Here's how the part is built. I have some questions about the finished solid (model axes, mm). A direction names the side the tool comes from. Round coordinates to 2 decimals unless told otherwise and drop trailing zeros. Order: outer loops, then holes, each group sorted by start corner. A loop starts at its lowest first (then second) coordinate and runs counter-clockwise, first axis right, second up. Notation, with made-up numbers: (44.25, 32.5) -> (51.25, 32.5) arc R19 cw to (51.25, 61.5) -> close; hole circle Ø8 at (-14.5, 86.5). An arc over 180 degrees is marked (long way). Use a Markdown table: item, result. Add a question column.
(1) On a 3-axis mill with a long thin cutter (end or side, diameter ignored), from which of +Z, -Z, +X, -X, +Y, -Y can I reach the whole of each face in a straight line? I mean faces 1 (the face through (0, 3.3, -5.2)), 2 (the face through (1, 3.4, -1)), 3 (the face through (1, 3, 1)). Say none if no direction works.
(2) I'm going to push flat-ended pins straight in: P1, Ø1.7, axis at x = -1, z = -6.5, coming from the -Y side; P2, Ø4, axis at x = 0, z = 0, coming from the +Y side; P3, Ø2.5, axis at x = -0.5, z = 0, coming from the -Y side; P4, Ø1.5, axis at y = 0.5, z = -5.5, coming from the -X side. Where does each tip first touch, or does it pass through?
(3) I want a section at B-B, the plane z = -6.8. Please give me the cut outline in (x, y), then the cut area to 3 significant figures.
(4) Thinking about a two-plate mould opening in Z: for faces 4 (the face through (0, 4.2, -6)), 5 (the face through (-1.45, 3.81, -1.88)), 6 (the face through (2.355, 3.287, -8.016)), which applies, pulls with the +Z half, pulls with the -Z half, needs draft (parallel to the pull), parting line crosses it, or undercut?
(5) I want a section at A-A, the plane z = -10.8. Please give me the cut outline in (x, y).
(6) If I drill on probe 1 along X at (y, z) = (3.25, 0) (3 decimals); probe 2 along X at (y, z) = (3.3, -10.8); probe 3 along Y at (x, z) = (1.25, -5), over which ranges is the centre line in solid material (lowest first)?
from build123d import *

# Parameters (mm, degrees)
SKETCH1_R           = 3.425
HUB_DEPTH           = 2.4
SKETCH2_R           = 0.4
BOSS_EXTRUDE2_DEPTH = 1.8
SKETCH3_R           = 2.375
CUT_EXTRUDE1_DEPTH  = 0.8
SKETCH4_R           = 1.2
CUT_EXTRUDE2_DEPTH  = 17.520612
CUT_EXTRUDE3_DEPTH  = 3
CIRPATTERN1_COUNT   = 36
SKETCH6_R           = 2.25
CUT_EXTRUDE4_DEPTH  = 3


with BuildPart() as part:
    # Sketch1 → HUB (new body)
    with BuildSketch(Plane(origin=(0, 0, 0), x_dir=(1, 0, 0), z_dir=(0, 1, 0))):
        with Locations(Location((0, 0, 0), (0, 0, 270))):
            Circle(SKETCH1_R)
    extrude(amount=HUB_DEPTH)

    # Sketch2 → Boss-Extrude2 (add)
    with BuildSketch(Plane(origin=(0, 2.4, 0), x_dir=(1, 0, 0), z_dir=(0, 1, 0))):
        with BuildLine():
            Line((-2.875, 1.861451), (-1.85, 14))
            add(Edge.make_bspline(
                [(-1.85, 14), (-1.761904, 15.043277), (-0.882336, 15.809649), (0.882387, 15.802355), (1.755744, 15.11622), (1.85, 14)],
                knots=[0, 0, 0, 0, 0.45, 0.55, 1, 1, 1, 1], degree=3))
            Line((1.85, 14), (2.875, 1.861451))
            ThreePointArc((2.875, 1.861451), (0, -3.425), (-2.875, 1.861451))
        make_face()
        with Locations(Location((0, 14.8, 0), (0, 0, 270))):
            Circle(SKETCH2_R, mode=Mode.SUBTRACT)
        with Locations(Location((0, 12.8, 0), (0, 0, 270))):
            Circle(SKETCH2_R, mode=Mode.SUBTRACT)
        with Locations(Location((0, 10.8, 0), (0, 0, 270))):
            Circle(SKETCH2_R, mode=Mode.SUBTRACT)
        with Locations(Location((0, 8.8, 0), (0, 0, 270))):
            Circle(SKETCH2_R, mode=Mode.SUBTRACT)
        with Locations(Location((0, 6.8, 0), (0, 0, 270))):
            Circle(SKETCH2_R, mode=Mode.SUBTRACT)
        with Locations(Location((0, 4.8, 0), (0, 0, 270))):
            Circle(SKETCH2_R, mode=Mode.SUBTRACT)
    extrude(amount=BOSS_EXTRUDE2_DEPTH)

    # Sketch3 → Cut-Extrude1 (cut)
    with BuildSketch(Plane(origin=(0, 4.2, 0), x_dir=(1, 0, 0), z_dir=(0, 1, 0))):
        with Locations(Location((0, 0, 0), (0, 0, 270))):
            Circle(SKETCH3_R)
    extrude(amount=-CUT_EXTRUDE1_DEPTH, mode=Mode.SUBTRACT)

    # Sketch4 → Cut-Extrude2 (cut, through all)
    with BuildSketch(Plane(origin=(0, 3.4, 0), x_dir=(1, 0, 0), z_dir=(0, 1, 0))):
        with Locations(Location((0, 0, 0), (0, 0, 270))):
            Circle(SKETCH4_R)
    extrude(amount=-CUT_EXTRUDE2_DEPTH, mode=Mode.SUBTRACT)

    # Sketch5 → Cut-Extrude3 (cut)
    with BuildSketch(Plane.XZ):
        with BuildLine():
            Line((0, 2.45), (-0.173437, 2.243305))
            ThreePointArc((-0.173437, 2.243305), (0, 2.25), (0.173437, 2.243305))
            Line((0.173437, 2.243305), (0, 2.45))
        make_face()
    cut_extrude3 = extrude(amount=-CUT_EXTRUDE3_DEPTH, mode=Mode.SUBTRACT)

    # CirPattern1: Cut-Extrude3 ×36 about axis
    cirpattern1_axis = Axis((0, 0, 0), (0, 1, 0))
    for i in range(1, CIRPATTERN1_COUNT):
        add(cut_extrude3.rotate(cirpattern1_axis, i * 360 / CIRPATTERN1_COUNT), mode=Mode.SUBTRACT)

    # Sketch6 → Cut-Extrude4 (cut)
    with BuildSketch(Plane.XZ):
        Circle(SKETCH6_R)
    extrude(amount=-CUT_EXTRUDE4_DEPTH, mode=Mode.SUBTRACT)


solid = part.part
Taken from the geometry:
| question | item | result |
|---|---|---|
| 1 | face 1 | +Y, -Y |
| 1 | face 2 | +Y |
| 1 | face 3 | -Y |
| 2 | P1 | stops at y = 2.4 |
| 2 | P2 | stops at y = 3.4 |
| 2 | P3 | stops at y = 3 |
| 2 | P4 | passes through |
| 3 | outline | (-2.46, 2.4) -> (-0.4, 2.4) -> (-0.4, 4.2) -> (-2.46, 4.2) -> close; (0.4, 2.4) -> (2.46, 2.4) -> (2.46, 4.2) -> (0.4, 4.2) -> close |
| 3 | area | 7.41 mm2 |
| 4 | face 4 | needs draft |
| 4 | face 5 | undercut |
| 4 | face 6 | pulls with the -Z half |
| 5 | outline | (-2.12, 2.4) -> (-0.4, 2.4) -> (-0.4, 4.2) -> (-2.12, 4.2) -> close; (0.4, 2.4) -> (2.12, 2.4) -> (2.12, 4.2) -> (0.4, 4.2) -> close |
| 6 | probe 1 | x = -3.425 to -1.2, 1.2 to 3.425 |
| 6 | probe 2 | x = -2.12 to -0.4, 0.4 to 2.12 |
| 6 | probe 3 | y = 2.4 to 4.2 |
